For this review, take the finished solid that the model builds, in its own axes (mm). A direction names the side the tool comes from. Coordinates: 2 decimals unless noted, no trailing zeros. Loops run counter-clockwise (first coordinate to the right, second up) from the corner with the lowest first, then second, coordinate; pieces in that order, holes last.
```python
from build123d import *

# Parameters (mm, degrees)
F3_DEPTH = 5
F4_R     = 2


with BuildPart() as f1:
    # F0 (on Front) → F1 (revolve)
    with BuildSketch(Plane.XZ):
        Polygon((0, 15), (0, 0), (2, 0), (2, 6), (4, 6), (4, 9), (4.5, 9), (4.5, 10), (4, 10), (4, 15), align=None)
    revolve(axis=Axis((0, 0, 7.5), (0, 0, -1)))

    # F2 (on face) → F3 (cut, through all)
    with BuildSketch(Plane.XY.offset(15)):
        with BuildLine():
            Line((-1, -3.8729833462), (-1, 3.8729833462))
            ThreePointArc((-1, 3.8729833462), (-4, 0), (-1, -3.8729833462))
        make_face()
        with BuildLine():
            ThreePointArc((4, 0), (3.1622776602, 2.4494897428), (1, 3.8729833462))
            Line((1, 3.8729833462), (1, -3.8729833462))
            ThreePointArc((1, -3.8729833462), (3.1622776602, -2.4494897428), (4, 0))
        make_face()
    extrude(amount=-F3_DEPTH, mode=Mode.SUBTRACT)

    # F4
    f4_edges = [f1.edges().sort_by_distance(p)[0] for p in [
        (0, -4, 15),
        (0, 4, 15),
    ]]
    fillet(f4_edges, radius=F4_R)


solid = f1.part
```
Q1. Machinability: for faces 4 (the face through (1, 0, 13)), 5 (the face through (0, -4, 12)), 6 (the face through (-0.867, 3.905, 7.521)), 7 (the face through (-1, 0, 13)), which of the approach directions +Z, -Z, +X, -X, +Y, -Y give a long, thin tool a straight path to every point of the face, cutting with its end or side? Answer none if there is none.
Q2. Consider section A-A (y = 0). State the section outline as (x, z) points, then the cut area to 3 significant figures.
Q3. For pin 1 Ø3 at (x, y) = (-1.5, -2) entering from +Z; pin 2 Ø2 at (x, y) = (2, -3.5) entering from -Z; pin 3 Ø4 at (x, z) = (2, 13) entering from +Y; pin 4 Ø1.5 at (y, z) = (-1.5, 4) entering from -X, all flat-tipped, find the tip position at first contact; note any pin that passes through.
Q4. Consider section B-B (x = -2.75). State the section outline as (y, z) points, then the cut area to 3 significant figures.
Q5. Consider section C-C (z = 2.5). State the section outline as (x, y) points.
Q6. Consider section D-D (y = -1.5). State the section outline as (x, z) points.
Q7. The part is to be moulded in two halves that separate along Y. For faces 1 (the face through (3, 3, 9)), 2 (the face through (0, 2, 3)), 3 (the face through (0, 4, 12)), say which applies: +Y half, -Y half, draft (parallel to the pull), parting line (faces both ways), or undercut.
Q8. Wall thickness on probe 1 along Z at (x, y) = (-1.25, -0.5); probe 2 along Z at (x, y) = (3, -2.5); probe 3 along X at (y, z) = (-1.5, 11.5): over which ranges is each line inside the solid? List them lowest first.
Model answer:
1. face 4: +Z, +X, +Y, -Y
1. face 5: +Z, -Y
1. face 6: -Z
1. face 7: +Z, -X, +Y, -Y
2. outline: (-4.5, 9) - (-4, 9) - (-4, 6) - (-2, 6) - (-2, 0) - (2, 0) - (2, 6) - (4, 6) - (4, 9) - (4.5, 9) - (4.5, 10) - (1, 10) - (1, 15) - (-1, 15) - (-1, 10) - (-4.5, 10) - close
2. area: 67.0 mm2
3. pin 1: stops at z = 15
3. pin 2: stops at z = 6
3. pin 3: stops at y = 4
3. pin 4: stops at x = -1.85
4. outline: (-3.56, 9) - (-2.9, 9) - (-2.9, 6) - (2.9, 6) - (2.9, 9) - (3.56, 9) - (3.56, 10) - (-3.56, 10) - close
4. area: 24.6 mm2
5. outline: circle Ø4 at (0, 0)
6. outline: (-4.24, 9) - (-3.71, 9) - (-3.71, 6) - (-1.32, 6) - (-1.32, 0) - (1.32, 0) - (1.32, 6) - (3.71, 6) - (3.71, 9) - (4.24, 9) - (4.24, 10) - (1, 10) - (1, 15) - (-1, 15) - (-1, 10) - (-4.24, 10) - close
7. face 1: draft
7. face 2: parting line
7. face 3: +Y half
8. probe 1: z = 0 to 10
8. probe 2: z = 6 to 10
8. probe 3: x = -1 to 1
